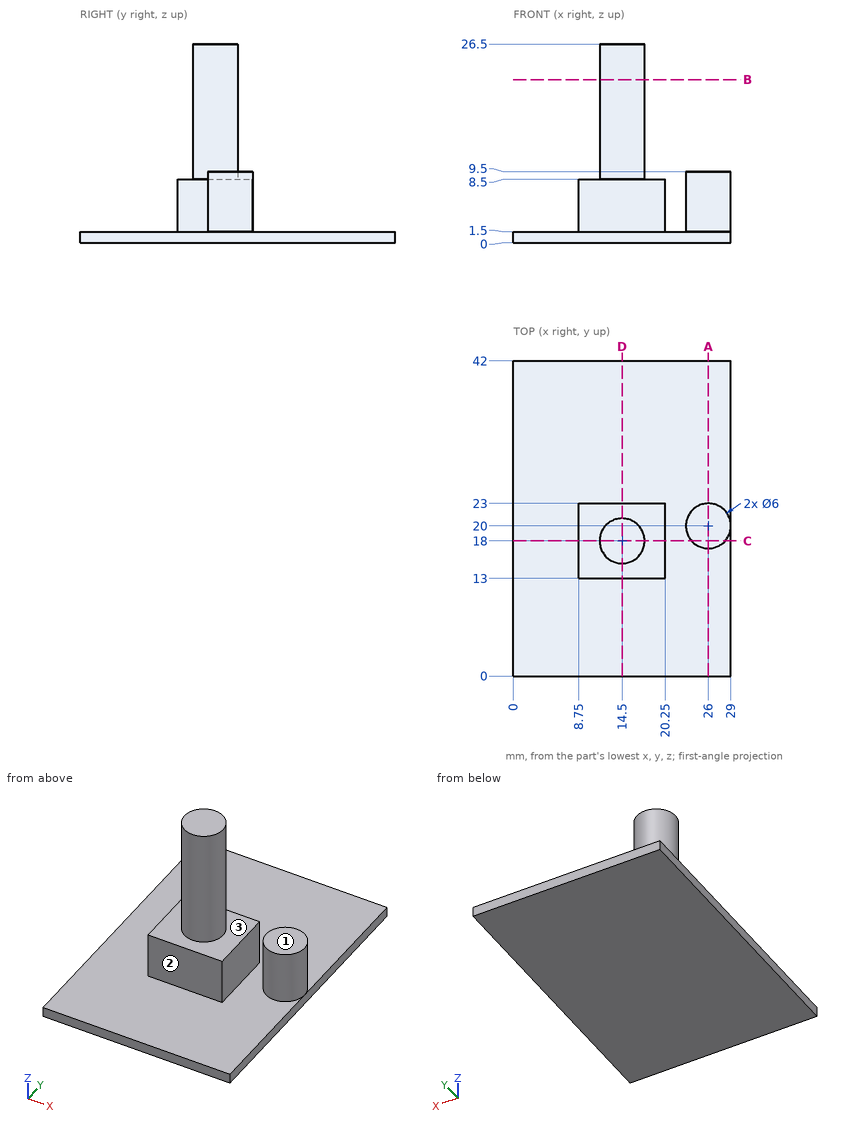
Geometry check sheet. Reference: drawing and pictorial views, mm from the part's lowest x, y, z. A direction names the side the tool comes from. Round coordinates to 2 decimals unless told otherwise and drop trailing zeros. Loops run counter-clockwise (first coordinate to the right, second up) from the corner with the lowest first, then second, coordinate; pieces in that order, holes last. Notation, with made-up numbers: (28, 24.25) -> (59, 24.25) arc R10 ccw to (59, 32.25) -> close; hole circle Ø11 at (53.5, 78.25). An arc over 180 degrees is marked (long way). Answer as a JSON object with one key per item and string values. Group by question number.
Item 1: Depth check by flat-ended pin: pin 1 Ø3.5 at (y, z) = (19.5, 6) entering from -X; pin 2 Ø7.5 at (x, z) = (16.5, 6.5) entering from -Y; pin 3 Ø3 at (x, z) = (11, 17.5) entering from +Y; pin 4 Ø12 at (x, y) = (17, 12) entering from +Z. Enter the tip coordinate at first touch or a pass-through.
Item 2: Cross-section at B-B, the plane z = 21.75. Record the cut outline in (x, y), plus the area to 3 significant figures.
Item 3: Cross-section at C-C, the plane y = 18. Record the cut outline in (x, z).
Item 4: Cross-section at A-A, the plane x = 26. Record the cut outline in (y, z), plus the area to 3 significant figures.
Item 5: Set-up check for the marked faces 1, 2 and 3: record each of +Z, -Z, +X, -X, +Y, -Y from which the full face is reachable in a straight line by a thin tool's end or side.
Item 6: Thickness scan on line 1 along Z through (x, y) = (2.5, 6); line 2 along X through (y, z) = (22.5, 6.75); line 3 along Y through (x, z) = (17, 4). Record the ranges inside material, lowest first.
Item 7: Cross-section at D-D, the plane x = 14.5. Record the cut outline in (y, z), plus the area to 3 significant figures.
Determined:
{
 "1": {"pin 1": "stops at x = 8.75", "pin 2": "stops at y = 13", "pin 3": "stops at y = 20.24", "pin 4": "stops at z = 26.5"},
 "2": {"outline": "circle Ø6 at (14.5, 18)", "area": "28.3 mm²"},
 "3": {"outline": "(0, 0) -> (29, 0) -> (29, 1.5) -> (28.24, 1.5) -> (28.24, 9.5) -> (23.76, 9.5) -> (23.76, 1.5) -> (20.25, 1.5) -> (20.25, 8.5) -> (17.5, 8.5) -> (17.5, 26.5) -> (11.5, 26.5) -> (11.5, 8.5) -> (8.75, 8.5) -> (8.75, 1.5) -> (0, 1.5) -> close"},
 "4": {"outline": "(0, 0) -> (42, 0) -> (42, 1.5) -> (23, 1.5) -> (23, 9.5) -> (17, 9.5) -> (17, 1.5) -> (0, 1.5) -> close", "area": "111 mm²"},
 "5": {"face 1": "+Z, +X, +Y, -Y", "face 2": "+Z, +X, -X, -Y", "face 3": "+Z"},
 "6": {"line 1": "z = 0 to 1.5", "line 2": "x = 8.75 to 20.25, 24.34 to 27.66", "line 3": "y = 13 to 23"},
 "7": {"outline": "(0, 0) -> (42, 0) -> (42, 1.5) -> (23, 1.5) -> (23, 8.5) -> (21, 8.5) -> (21, 26.5) -> (15, 26.5) -> (15, 8.5) -> (13, 8.5) -> (13, 1.5) -> (0, 1.5) -> close", "area": "241 mm²"}
}
